```python
from build123d import *

# Parameters (mm, degrees)
F0_R     = 35
F0_R_2   = 2.55
F1_DEPTH = 5
F3_DEPTH = 10


with BuildPart() as f1:
    # F0 (on Top) → F1 (new body)
    with BuildSketch(Plane.XY):
        Circle(F0_R)
        Circle(F0_R_2, mode=Mode.SUBTRACT)
    extrude(amount=F1_DEPTH)

    # F2 (on face) → F3 (join)
    with BuildSketch(Plane.XY.offset(5)):
        Polygon((1.943101, -23.666137), (0, -18.927574), (0, -28.927574), (2.5, -28.927574), align=None)
    extrude(amount=F3_DEPTH)


solid = f1.part
```
The listing builds one solid part. Answer for the finished solid, in the listing's coordinates (mm). A direction names the side the tool comes from. Give positions to 0.01 mm unless a question says otherwise; leave off trailing zeros. Order: outer loops, then holes, each group sorted by start corner. A loop starts at its lowest first (then second) coordinate and runs counter-clockwise, first axis right, second up. Notation, with made-up numbers: M -31,8.5 L -18,8.5 A24 ccw -18,22.5 Z; hole C -31.75,86.25 d11. An arc over 180 degrees is marked long. Put each result on its own line as item: value. Start each with the question number.
Item 1: For a pull along Z with two mould halves and no side action, classify faces 1 (the face through (0, -7, 0)), 2 (the face through (1, -25, 15)), 3 (the face through (-28, -21, 2)) as +Z half, -Z half, draft (parallel to the pull), parting line (faces both ways), or undercut.
Item 2: Which of the six approach directions +Z, -Z, +X, -X, +Y, -Y give full straight-line access (tool end or side, diameter ignored) to faces 4 (the face through (1, -28.928, 10)), 5 (the face through (1.18, -2.26, 2.46)), 6 (the face through (0, -24, 10)), 7 (the face through (0.985, -21.33, 9.93))?
Item 3: Find the intervals of material crossed by line 1 along Y through (x, z) = (0, 3); line 2 along Z through (x, y) = (0, -7.5); line 3 along X through (y, z) = (-31, 1), in increasing order.
Item 4: The part is cut by section C-C, the plane y = -27. Determine the outline of the cut face in (x, z), and give its area (3 significant figures).
Item 5: The part is cut by section B-B, the plane z = 3.75. Determine the outline of the cut face in (x, y), and give its area (3 significant figures).
Item 6: The part is cut by section D-D, the plane z = 12.5. Determine the outline of the cut face in (x, y), and give its area (3 significant figures).
Item 7: The part is cut by section A-A, the plane y = 0. Determine the outline of the cut face in (x, z), and give its area (4 significant figures).
Item 8: Flat-ended cylindrical pins translate along their axes: P1, Ø1.2, axis at x = 1.5, z = 11, coming from the -Y side; P2, Ø12, axis at x = 22.5, y = -5.5, coming from the +Z side; P3, Ø1, axis at y = 14, z = 4.5, coming from the -X side; P4, Ø4.5, axis at x = 0, y = 0, coming from the -Z side. Find the tip coordinate at first contact, or state that the pin passes through.
Answer key:
1. face 1: -Z half
1. face 2: +Z half
1. face 3: draft
2. face 4: +Z, +X, -X, -Y
2. face 5: +Z, -Z
2. face 6: +Z, -X, +Y, -Y
2. face 7: +Z, +X, +Y
3. line 1: y = -35 to -2.55, 2.55 to 35
3. line 2: z = 0 to 5
3. line 3: x = -16.25 to 16.25
4. outline: M -22.27,0 L 22.27,0 L 22.27,5 L 2.3,5 L 2.3,15 L 0,15 L 0,5 L -22.27,5 Z
4. area: 246 mm²
5. outline: C 0,0 d70; hole C 0,0 d5.1
5. area: 3,830 mm²
6. outline: M 0,-28.93 L 2.5,-28.93 L 1.94,-23.67 L 0,-18.93 Z
6. area: 16.3 mm²
7. outline: M -35,0 L -2.55,0 L -2.55,5 L -35,5 Z; M 2.55,0 L 35,0 L 35,5 L 2.55,5 Z
7. area: 324.5 mm²
8. P1: stops at y = -28.93
8. P2: stops at z = 5
8. P3: stops at x = -32.29
8. P4: passes through
